The listing builds one solid part. Answer for the finished solid, in the listing's coordinates (mm). A direction names the side the tool comes from. Give positions to 0.01 mm unless a question says otherwise; leave off trailing zeros. Order: outer loops, then holes, each group sorted by start corner. A loop starts at its lowest first (then second) coordinate and runs counter-clockwise, first axis right, second up. Notation, with made-up numbers: (49.25, -7) - (62.25, -7) arc R20 ccw to (62.25, 19) - close; hole circle Ø4 at (-6.5, -30). An arc over 180 degrees is marked (long way). Answer as a JSON object with one key per item and string values. Group by question number.
Q1. A cutting plane is placed at B-B, the plane y = 4.25. Give the vertices of the cut face in (x, z), and give its area (3 significant figures).
Q2. A cutting plane is placed at A-A, the plane z = 0. Give the vertices of the cut face in (x, y).
Q3. For faces 1 (the face through (38.944, 10.14, -27.269)), 2 (the face through (0, 18, 24)), 3 (the face through (-5.24, 7.82, 26.96)), 4 (the face through (24, 0, 19)), 5 (the face through (38.944, 10.14, 27.269)), determine the directions among +Z, -Z, +X, -X, +Y, -Y from which every point of the face is accessible in a straight line to the end or side of a thin tool.
Q4. A cutting plane is placed at D-D, the plane y = 18.5. Give the vertices of the cut face in (x, z), and give its area (3 significant figures).
Q5. Consider line 1 (X direction, y = 13.75, z = 18); line 2 (X direction, y = 15.75, z = 21.5); line 3 (X direction, y = 1, z = -11.5). Determine where each line is inside the solid, lowest interval first.
Q6. The mould has two halves that part along X. Classify faces 6 (the face through (5.14, 14.85, 21.096)), 7 (the face through (-3.775, 18.749, -11.986)), 8 (the face through (50.534, 10, 0)), 9 (the face through (22, 20, 0)): released by +X, released by -X, zero draft, split by the parting line, or undercut.
Q7. A cutting plane is placed at C-C, the plane x = 0. Give the vertices of the cut face in (y, z), and give its area (3 significant figures).
Q8. Given pin 1 (4 mm diameter, centred on y = 16.5, z = 4.5, fed in from -X); pin 2 (1 mm diameter, centred on x = 14, y = 10, fed in from -Z); pin 3 (2 mm diameter, centred on x = -14.5, z = -12, fed in from -Y), each flat-ended and moving along its own axis, determine where each tip first touches the part or whether it passes through.
from build123d import *

# Parameters (mm, degrees)
REVOLVE2_ANGLE          = 70
CUT_EXTRUDE1_DEPTH      = 78.096292231
CUT_EXTRUDE1_DEPTH_BACK = 78.096292231
SKETCH4_W               = 54.680091263
SKETCH4_H               = 66.719762054
SKETCH5_R               = 6
CUT_EXTRUDE2_DEPTH      = 40
CUT_REVOLVE1_ANGLE      = 22


with BuildPart() as part:
    # Sketch1 → Revolve1 (revolve)
    with BuildSketch(Plane(origin=(0, 0, 0), x_dir=(0, 0, -1), z_dir=(1, 0, 0))):
        Polygon((11.5, 20), (28.55, 0), (41.690609765, 0), (24.640609765, 20), align=None)
    revolve(axis=Axis((0, 0, 0), (0, 1, 0)))

    # Sketch3 → Revolve2 (revolve, symmetric)
    with BuildSketch(Plane.XY) as revolve2_sk:
        Polygon((24.640609765, 20), (61.690609765, 20), (61.690609765, 0), (41.690609765, 0), align=None)
    revolve(axis=Axis((0, 0, 0), (0, 1, 0)), revolution_arc=REVOLVE2_ANGLE / 2)
    revolve(revolve2_sk.sketch, axis=Axis((0, 0, 0), (0, -1, 0)), revolution_arc=REVOLVE2_ANGLE / 2)

    # Sketch4 → Cut-Extrude1 (cut, two sides: drawn at the far end of the back side and taken through both)
    with BuildSketch(Plane.XY.offset(-CUT_EXTRUDE1_DEPTH_BACK)):
        with Locations((77.874034735, 12.769248077)):
            Rectangle(SKETCH4_W, SKETCH4_H)
    extrude(amount=CUT_EXTRUDE1_DEPTH + CUT_EXTRUDE1_DEPTH_BACK, mode=Mode.SUBTRACT)

    # Sketch5 → Cut-Extrude2 (cut)
    with BuildSketch(Plane(origin=(0, 0, 0), x_dir=(1, 0, 0), z_dir=(0, 1, 0))):
        with Locations(Location((0, -18, 0), (0, 0, 251.911143057))):
            Circle(SKETCH5_R)
    extrude(amount=CUT_EXTRUDE2_DEPTH, mode=Mode.SUBTRACT)

    # Sketch7 → Cut-Revolve1 (revolve, symmetric, cut)
    with BuildSketch(Plane(origin=(0, 0, 0), x_dir=(0, 0, -1), z_dir=(1, 0, 0))) as cut_revolve1_sk:
        Polygon((-43.736107379, -8.562897575), (-24, 14.94597317), (-24, 20), (-18.43156125, 20), (-18.70488034, 12.563709667), (-17.388176204, -8.562897575), align=None)
    revolve(axis=Axis((0, 0, 0), (0, 1, 0)), revolution_arc=CUT_REVOLVE1_ANGLE / 2, mode=Mode.SUBTRACT)
    revolve(cut_revolve1_sk.sketch, axis=Axis((0, 0, 0), (0, -1, 0)), revolution_arc=CUT_REVOLVE1_ANGLE / 2, mode=Mode.SUBTRACT)


solid = part.part
Reply:
{
 "1": {"outline": "(31.18, -21.83) - (50.53, -35.38) - (50.53, 35.38) - (31.18, 21.83) arc R38.07 ccw (long way) to start; hole (-6.29, 32.37) - (-4.76, 24.47) arc R24.93 ccw (long way) to (4.76, 24.47) - (6.29, 32.37) arc R32.98 ccw to start", "area": "3,410 mm^2"},
 "2": {"outline": "(-41.69, 0) - (-28.55, 0) - (-11.5, 20) - (-24.64, 20) - close; (11.5, 20) - (28.55, 0) - (50.53, 0) - (50.53, 20) - close"},
 "3": {"face 1": "-Z, +Y", "face 2": "+Y, -Y", "face 3": "-Y", "face 4": "+Z, -Z, +X, -X, -Y", "face 5": "+Z, +Y"},
 "4": {"outline": "(21.23, -14.87) - (50.53, -35.38) - (50.53, 35.38) - (21.23, 14.87) arc R25.92 ccw (long way) to start; hole (-4.58, 23.56) - (-4.31, 22.17) arc R6 ccw to (-2.48, 12.54) arc R12.78 ccw (long way) to (2.48, 12.54) arc R6 ccw to (4.31, 22.17) - (4.58, 23.56) arc R24 ccw to start", "area": "2,860 mm^2"},
 "5": {"line 1": "x = -23.96 to -6, 6 to 23.96, 25.71 to 50.53", "line 2": "x = -18.35 to -4.87, 4.87 to 18.35, 30.71 to 50.53", "line 3": "x = -39.19 to -25.2, 25.2 to 50.53"},
 "6": {"face 6": "undercut", "face 7": "undercut", "face 8": "released by +X", "face 9": "zero draft"},
 "7": {"outline": "(0, -41.69) - (20, -24.64) - (20, -11.5) - (0, -28.55) - close; (0, 36.55) - (14.95, 24) - (20, 24) - (20, 24.64) - (0, 41.69) - close; (19.41, 12) - (20, 11.5) - (20, 12) - close", "area": "353 mm^2"},
 "8": {"pin 1": "stops at x = -29.01", "pin 2": "stops at z = -30.59", "pin 3": "stops at y = 10.24"}
}
